The listing builds one solid part. Answer for the finished solid, in the listing's coordinates (mm). Coordinates: 2 decimals unless noted, no trailing zeros. Order: outer loops, then holes, each group sorted by start corner. A loop starts at its lowest first (then second) coordinate and runs counter-clockwise, first axis right, second up. Notation, with made-up numbers: (46.5, -19) -> (101.5, -19) arc R11 ccw to (101.5, -7) -> close; hole circle Ø7 at (-15, -7.5). An arc over 180 degrees is marked (long way). Return JSON: item names as keys, results as strings.
Autodesk Inventor part; units mm, degrees
ref_plane "YZ Plane" through (0, 0, 0) normal (1, 0, 0) x (0, 1, 0)
ref_plane "XZ Plane" through (0, 0, 0) normal (0, 1, 0) x (-1, 0, 0)
ref_plane "XY Plane" through (0, 0, 0) normal (0, 0, 1) x (1, 0, 0)
sketch "Sketch1" plane through (0, 0, 0) normal (1, 0, 0) x (0, 1, 0)
  line L0 (0, 0) -> (120, 0)
  line L1 (120, 0) -> (120, -99)
  line L2 (120, -99) -> (0, -99)
  line L3 (0, -99) -> (0, 0)
  dimension "d0" = 120
  dimension "d1" = 99
extrude "Extrusion1" add sketch "Sketch1" along normal blind 6
sketch "Sketch2" plane through (6, 0, 0) normal (1, 0, 0) x (0, 0, -1)
  line L0 (0, 120) -> (0, 0)
  line L1 (0, 0) -> (99, 0)
  line L2 (99, 0) -> (99, 120)
  line L3 (99, 120) -> (0, 120)
  line L4 (0, 120) -> (0, 0)
  line L5 (0, 15) -> (5.75, 15)
  line L6 (5.75, 15) -> (5.75, 45)
  line L7 (5.75, 45) -> (0, 45)
  line L8 (0, 45) -> (0, 15)
  line L9 (0, 75) -> (5.75, 75)
  line L10 (5.75, 75) -> (5.75, 105)
  line L11 (5.75, 105) -> (0, 105)
  line L12 (0, 105) -> (0, 75)
  line L13 (99, 15) -> (93.25, 15)
  line L14 (93.25, 15) -> (93.25, 45)
  line L15 (93.25, 45) -> (99, 45)
  line L16 (99, 45) -> (99, 15)
  line L17 (99, 75) -> (93.25, 75)
  line L18 (93.25, 75) -> (93.25, 105)
  line L19 (93.25, 105) -> (99, 105)
  line L20 (99, 105) -> (99, 75)
  line L21 (-12.0657, 60) -> (104.2665, 60)
  line L22 (99, 120) -> (0, 120)
  dimension "d5" = 5.75
  dimension "d6" = 5.75
  dimension "d8" = 30
  dimension "d9" = 30
  dimension "d22" = 60
  dimension "d23" = 15
  dimension "d24" = 15
extrude "Extrusion2" cut sketch "Sketch2" against normal up to next contours L11 L10 L9 L0 | L2 L17 L18 L19 | L7 L6 L5 L0 | L2 L13 L14 L15
sketch "Sketch3" plane through (6, 0, 0) normal (1, 0, 0) x (0, 0, -1)
  circle A0 centre (79, 10) radius 2.3
  circle A1 centre (79, 110) radius 2.3
  line L0 (99, 105) -> (99, 120)
  line L1 (99, 120) -> (0, 120)
  line L2 (99, 0) -> (99, 15)
  line L3 (0, 0) -> (99, 0)
  dimension "d13" = 20
  dimension "d14" = 10
  dimension "d15" = 4.6
  dimension "d17" = 10
  dimension "d18" = 20
  dimension "d19" = 4.6
extrude "Extrusion3" cut sketch "Sketch3" against normal up to next
sketch "Sketch4" plane through (6, 0, 0) normal (1, 0, 0) x (0, 0, -1)
  circle A0 centre (79, 10) radius 2.3
  circle A1 centre (79, 110) radius 2.3
  line L0 (5.75, 75) -> (0, 75)
  line L1 (0, 75) -> (0, 45)
  line L2 (0, 45) -> (5.75, 45)
  line L3 (5.75, 45) -> (5.75, 15)
  line L4 (5.75, 15) -> (0, 15)
  line L5 (0, 15) -> (0, 0)
  line L6 (0, 0) -> (99, 0)
  line L7 (99, 0) -> (99, 15)
  line L8 (99, 15) -> (93.25, 15)
  line L9 (93.25, 15) -> (93.25, 45)
  line L10 (93.25, 45) -> (99, 45)
  line L11 (99, 45) -> (99, 75)
  line L12 (99, 75) -> (93.25, 75)
  line L13 (93.25, 75) -> (93.25, 105)
  line L14 (93.25, 105) -> (99, 105)
  line L15 (99, 105) -> (99, 120)
  line L16 (99, 120) -> (0, 120)
  line L17 (0, 120) -> (0, 105)
  line L18 (0, 105) -> (5.75, 105)
  line L19 (5.75, 105) -> (5.75, 75)
  circle A2 centre (33.095, 103.598) radius 1.5 construction
  circle A3 centre (33.095, 93.242) radius 1.5 construction
  arc A4 (22.095, 105.098) -> (22.095, 102.098) centre (22.095, 103.598) ccw
  arc A5 (38.095, 102.098) -> (38.095, 105.098) centre (38.095, 103.598) ccw
  arc A6 (22.095, 94.742) -> (22.095, 91.742) centre (22.095, 93.242) ccw
  arc A7 (38.095, 91.742) -> (38.095, 94.742) centre (38.095, 93.242) ccw
  line L20 (22.095, 91.742) -> (38.095, 91.742)
  line L21 (22.095, 94.742) -> (38.095, 94.742)
  line L22 (22.095, 102.098) -> (38.095, 102.098)
  line L23 (22.095, 105.098) -> (38.095, 105.098)
  dimension "d25" = 3
  dimension "d26" = 3
  dimension "d27" = 10.356
  dimension "d28" = 16.402
  dimension "d29" = 65.905
  dimension "d30" = 3
  dimension "d31" = 3
  dimension "d32" = 3
  dimension "d33" = 3
  dimension "d34" = 16
  dimension "d35" = 16
  dimension "d36" = 11
  dimension "d37" = 11
extrude "Extrusion4" cut sketch "Sketch4" against normal blind 10 contours L23 A5 L22 A4 | L21 A7 L20 A6
equation "\"d26\" = d25"
equation "\"d30\" = d25"
equation "\"d31\" = d25"
equation "\"d32\" = d25"
equation "\"d33\" = d25"
properties part number "SideLeft"
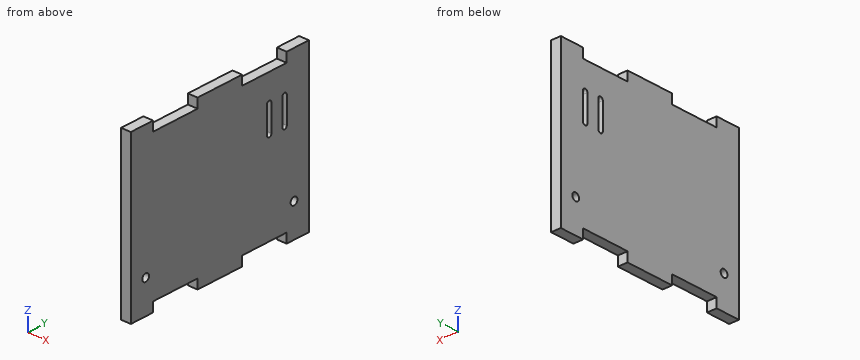
1. The part is cut by section B-B on y = 10. Give the vertices of the cut face in (x, z).
Answer block:
{"outline": "(0, -99) -> (6, -99) -> (6, -81.3) -> (0, -81.3) -> close; (0, -76.7) -> (6, -76.7) -> (6, 0) -> (0, 0) -> close"}
2. The part is cut by section A-A on z = -79. Give the vertices of the cut face in (x, y), and give its area (3 significant figures).
Answer block:
{"outline": "(0, 0) -> (6, 0) -> (6, 7.7) -> (0, 7.7) -> close; (0, 12.3) -> (6, 12.3) -> (6, 107.7) -> (0, 107.7) -> close; (0, 112.3) -> (6, 112.3) -> (6, 120) -> (0, 120) -> close", "area": "665 mm2"}
3. The part is cut by section C-C on x = 3.95. Give the number of separate pieces and of enclosed holes in the cut face, and give its area (3 significant figures).
Answer block:
{"separate pieces": "1", "enclosed holes": "4", "area": "11,000 mm2"}
4. Consider line 1 (Y direction, x = 4.35, z = -79); line 2 (Y direction, x = 4.75, z = -29); line 3 (Z direction, x = 4.75, y = 88). Determine where each line is inside the solid, lowest interval first. Write a range as from..to.
Answer block:
{"line 1": "y = 0..7.7, 12.3..107.7, 112.3..120", "line 2": "y = 0..91.74, 94.74..102.1, 105.1..120", "line 3": "z = -93.25..-5.75"}
5. Each of these flat-tipped pins is pushed along its axis until it touches: pin 1 Ø3 at (x, y) = (4.5, 93.5) entering from -Z; pin 2 Ø1.5 at (x, y) = (4, 42) entering from +Z. Where does it stop, or does it pass through?
Answer block:
{"pin 1": "stops at z = -93.25", "pin 2": "stops at z = -5.75"}
6. The part is cut by section D-D on y = 77. Give the vertices of the cut face in (x, z), and give its area (3 significant figures).
Answer block:
{"outline": "(0, -93.25) -> (6, -93.25) -> (6, -5.75) -> (0, -5.75) -> close", "area": "525 mm2"}
